The listing builds one solid part. Answer for the finished solid, in the listing's coordinates (mm). Give positions to 0.01 mm unless a question says otherwise; leave off trailing zeros. Loops run counter-clockwise (first coordinate to the right, second up) from the corner with the lowest first, then second, coordinate; pieces in that order, holes last. Notation, with made-up numbers: M 86,56 L 93,56 A26 cw 93,76 Z; hole C 25,53.5 d7. An arc over 180 degrees is marked long. One line per item, written item: value. Start each with the question number.
Q1. Consider L1, parallel to X at y = -51, z = 3; L2, parallel to Y at x = -20, z = 5.5; L3, parallel to Z at x = 169, y = -46.5. Determine where each line is inside the solid, lowest interval first.
Q2. A cutting plane is placed at C-C, the plane y = 37. Determine the outline of the cut face in (x, z).
Q3. The mould has two halves that part along X. Classify faces 1 (the flat face through (-1, 75.743, 3)), 2 (the flat face through (0, 101, 8.255)), 3 (the flat face through (-199.578, -2, 3)), 4 (the flat face through (199.578, -2, 3)): +X half, -X half, draft (parallel to the pull), parting line (faces both ways), or undercut.
Q4. A cutting plane is placed at A-A, the plane x = -62. Determine the outline of the cut face in (y, z), and give its area (3 significant figures).
Q5. Flat-ended cylindrical pins translate along their axes: pin 1 (1 mm diameter, centred on x = 7, z = 7.5, fed in from +Y); pin 2 (12 mm diameter, centred on x = 65.5, y = -75, fed in from +Z); pin 3 (2 mm diameter, centred on x = 183, z = 7.5, fed in from +Y). Find the tip coordinate at first contact, or state that the pin passes through.
Q6. A cutting plane is placed at B-B, the plane z = 3.75. Determine the outline of the cut face in (x, y), and give its area (3 significant figures).
Q7. A cutting plane is placed at D-D, the plane x = 153. Determine the outline of the cut face in (y, z) (3 decimals).
from build123d import *

# Parameters (mm, degrees)
F0_W     = 399.155342
F0_H     = 313.535798
F0_W_2   = 153.0096
F0_H_2   = 151.4856
F1_DEPTH = 6.35
F2_W     = 50.8
F2_H     = 50.8
F3_DEPTH = 1.905


with BuildPart() as f1:
    # F0 (on Top) → F1 (new body)
    with BuildSketch(Plane.XY):
        Rectangle(F0_W, F0_H)
        Rectangle(F0_W_2, F0_H_2, mode=Mode.SUBTRACT)
    extrude(amount=F1_DEPTH)

    # F2 (on face) → F3 (join)
    with BuildSketch(Plane.XY.offset(6.35)):
        with Locations((-174.177671, -105.287043)):
            Rectangle(F2_W, F2_H)
        with Locations((-174.177671, 81.533401)):
            Rectangle(F2_W, F2_H)
        with Locations((0.267005, 101.1428)):
            Rectangle(F2_W, F2_H)
        with Locations((174.177671, 103.394294)):
            Rectangle(F2_W, F2_H)
        with Locations((174.177671, -104.648051)):
            Rectangle(F2_W, F2_H)
    extrude(amount=F3_DEPTH)


solid = f1.part
Answer block:
1. L1: -199.58 to -76.5, 76.5 to 199.58
1. L2: -156.77 to -75.74, 75.74 to 156.77
1. L3: 0 to 6.35
2. outline: M -199.58,0 L -76.5,0 L -76.5,6.35 L -199.58,6.35 Z; M 76.5,0 L 199.58,0 L 199.58,6.35 L 76.5,6.35 Z
3. face 1: undercut
3. face 2: draft
3. face 3: -X half
3. face 4: +X half
4. outline: M -156.77,0 L -75.74,0 L -75.74,6.35 L -156.77,6.35 Z; M 75.74,0 L 156.77,0 L 156.77,6.35 L 75.74,6.35 Z
4. area: 1,030 mm^2
5. pin 1: y = 126.54
5. pin 2: z = 6.35
5. pin 3: y = 128.79
6. outline: M -199.58,-156.77 L 199.58,-156.77 L 199.58,156.77 L -199.58,156.77 Z; hole M -76.5,-75.74 L 76.5,-75.74 L 76.5,75.74 L -76.5,75.74 Z
6. area: 102,000 mm^2
7. outline: M -156.768,0 L 156.768,0 L 156.768,6.35 L 128.794,6.35 L 128.794,8.255 L 77.994,8.255 L 77.994,6.35 L -79.248,6.35 L -79.248,8.255 L -130.048,8.255 L -130.048,6.35 L -156.768,6.35 Z
